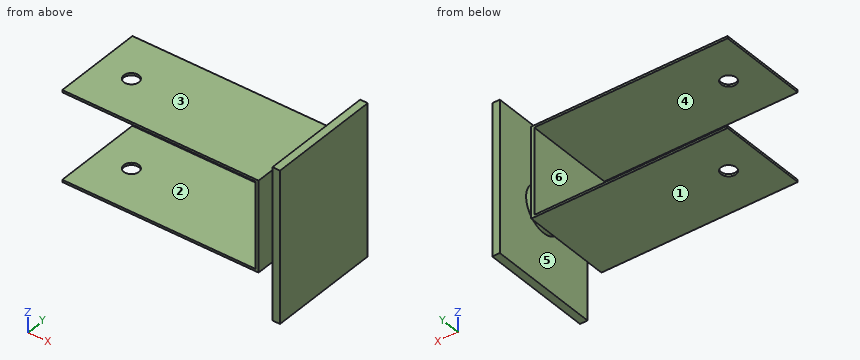
```python
from build123d import *

# Parameters (mm, degrees)
RESSALTO_EXTRUS_O1_DEPTH   = 60
CORTE_EXTRUS_O1_DEPTH      = 148.170653102
CORTE_EXTRUS_O1_DEPTH_BACK = 148.170653102
CORTE_EXTRUS_O2_DEPTH      = 148.170653102
CORTE_EXTRUS_O2_DEPTH_BACK = 148.170653102
ESBO_O5_W                  = 126
ESBO_O5_H                  = 57
ESBO_O6_W                  = 57
ESBO_O6_H                  = 60
CORTE_EXTRUS_O3_DEPTH      = 57
CORTE_EXTRUS_O4_DEPTH      = 148.170653102
CORTE_EXTRUS_O4_DEPTH_BACK = 57
ESBO_O7_R                  = 5
CORTE_EXTRUS_O5_DEPTH      = 148.170653102
CORTE_EXTRUS_O5_DEPTH_BACK = 148.170653102
ESBO_O8_W                  = 65.993133921
ESBO_O8_H                  = 60
ESBO_O13_R                 = 15
RESSALTO_EXTRUS_O2_DEPTH   = 15
ESBO_O14_W                 = 100
ESBO_O14_H                 = 75
RESSALTO_EXTRUS_O3_DEPTH   = 5


with BuildPart() as part:
    # Esboço1 → Ressalto-extrusão1 (new body)
    with BuildSketch(Plane.XY):
        with BuildLine():
            Line((65, 30), (-65, 30))
            Line((-65, 30), (-65, -30))
            Line((-65, -30), (65, -30))
            ThreePointArc((65, -30), (101.246012625, -22.148036763), (130.993133921, 0))
            ThreePointArc((130.993133921, 0), (101.246012625, 22.148036763), (65, 30))
        make_face()
    extrude(amount=RESSALTO_EXTRUS_O1_DEPTH)

    # Esboço3 → Corte-extrusão1 (cut, two sides: drawn at the far end of the back side and taken through both)
    with BuildSketch(Plane.XY.offset(-CORTE_EXTRUS_O1_DEPTH_BACK)):
        with BuildLine():
            Line((65, 25), (65, -25))
            ThreePointArc((65, -25), (88.305470739, -18.221231084), (104.339291624, 0))
            ThreePointArc((104.339291624, 0), (88.305470739, 18.221231084), (65, 25))
        make_face()
    extrude(amount=CORTE_EXTRUS_O1_DEPTH + CORTE_EXTRUS_O1_DEPTH_BACK, mode=Mode.SUBTRACT)

    # Esboço5 → Corte-extrusão2 (cut, two sides: drawn at the far end of the back side and taken through both)
    with BuildSketch(Plane(origin=(0, 0, 0), x_dir=(1, 0, 0), z_dir=(0, 1, 0)).offset(-CORTE_EXTRUS_O2_DEPTH_BACK)):
        with Locations((0, -30)):
            Rectangle(ESBO_O5_W, ESBO_O5_H)
    extrude(amount=CORTE_EXTRUS_O2_DEPTH + CORTE_EXTRUS_O2_DEPTH_BACK, mode=Mode.SUBTRACT)

    # Esboço6 → Corte-extrusão3 (cut)
    with BuildSketch(Plane(origin=(-63, 0, 0), x_dir=(0, 0, -1), z_dir=(1, 0, 0))):
        with Locations((-30, 0)):
            Rectangle(ESBO_O6_W, ESBO_O6_H)
    extrude(amount=-CORTE_EXTRUS_O3_DEPTH, mode=Mode.SUBTRACT)

    # Esboço7 → Corte-extrusão4 (cut, two sides: drawn at the far end of the back side and taken through both)
    with BuildSketch(Plane.XY.offset(-CORTE_EXTRUS_O4_DEPTH_BACK)):
        with Locations((-42.467037106, 0)):
            Circle(ESBO_O7_R)
    extrude(amount=CORTE_EXTRUS_O4_DEPTH + CORTE_EXTRUS_O4_DEPTH_BACK, mode=Mode.SUBTRACT)

    # Esboço8 → Corte-extrusão5 (cut, two sides: drawn at the far end of the back side and taken through both)
    with BuildSketch(Plane(origin=(0, 0, 0), x_dir=(1, 0, 0), z_dir=(0, 1, 0)).offset(-CORTE_EXTRUS_O5_DEPTH_BACK)):
        with Locations((97.996566961, -30)):
            Rectangle(ESBO_O8_W, ESBO_O8_H)
    extrude(amount=CORTE_EXTRUS_O5_DEPTH + CORTE_EXTRUS_O5_DEPTH_BACK, mode=Mode.SUBTRACT)

    # Esboço13 → Ressalto-extrusão2 (add)
    with BuildSketch(Plane(origin=(65, 0, 0), x_dir=(0, 0, -1), z_dir=(1, 0, 0))):
        with Locations((-30, 0)):
            Circle(ESBO_O13_R)
    extrude(amount=RESSALTO_EXTRUS_O2_DEPTH)

    # Esboço14 → Ressalto-extrusão3 (add)
    with BuildSketch(Plane(origin=(80, 0, 0), x_dir=(0, 0, -1), z_dir=(1, 0, 0))):
        with Locations((-30, 0)):
            Rectangle(ESBO_O14_W, ESBO_O14_H)
    extrude(amount=RESSALTO_EXTRUS_O3_DEPTH)


solid = part.part
```
Read the model definition and answer for the solid it produces. Units are mm, in the model's axes. Face numbers are marked on the shaded views. A direction names the side the tool comes from. Coordinates: 2 decimals unless noted, no trailing zeros. Write each loop counter-clockwise with the first axis right and the second up, starting at its lowest first coordinate (ties: lowest second). Pieces come first, ordered by that corner, then holes. Notation, with made-up numbers: (62.25, 8.5) -> (113.25, 8.5) arc R15 ccw to (113.25, 15.5) -> close; hole circle Ø2 at (69, 85). An arc over 180 degrees is marked (long way). Return JSON: item names as keys, results as strings.
1. Find the intervals of material crossed by line 1 along X through (y, z) = (0, 1); line 2 along Z through (x, y) = (15, -20); line 3 along X through (y, z) = (10, 18), in increasing order. Write a range as from..to.
Found:
{"line 1": "-65..-47.47, -37.47..65, 80..85", "line 2": "0..1.5, 58.5..60", "line 3": "63..65, 80..85"}
2. A tool of negligible diameter and unlimited length cuts with its end or side. For the marked faces 1, 2 and 3, from which of +Z, -Z, +X, -X, +Y, -Y can it reach the whole face along a straight path? Write none if from no direction.
Found:
{"face 1": "-Z, -X, +Y, -Y", "face 2": "-X, +Y, -Y", "face 3": "+Z, -X, +Y, -Y"}
3. A cutting plane is placed at A-A (z = 55). Determine the outline of the cut face in (x, y).
Found:
{"outline": "(63, -30) -> (65, -30) -> (65, 30) -> (63, 30) -> close; (80, -37.5) -> (85, -37.5) -> (85, 37.5) -> (80, 37.5) -> close"}
4. Determine the mould class of the marked faces 4, 5 and 6 for opening direction X: pulls with the +X half, pulls with the -X half, needs draft (parallel to the pull), parting line crosses it, or undercut.
Found:
{"face 4": "needs draft", "face 5": "undercut", "face 6": "pulls with the -X half"}
5. Each of these flat-tipped pins is pushed along its axis until it touches: P1, Ø1, axis at x = -28.5, y = -23, coming from the -Z side; P2, Ø12, axis at y = -7.5, z = 45, coming from the -X side; P3, Ø3, axis at x = 22, y = -25, coming from the +Z side. Where does it stop, or does it pass through?
Found:
{"P1": "z = 0", "P2": "x = 63", "P3": "z = 60"}
6. A cutting plane is placed at B-B (y = 0). Determine the outline of the cut face in (x, z).
Found:
{"outline": "(-65, 0) -> (-47.47, 0) -> (-47.47, 1.5) -> (-65, 1.5) -> close; (-65, 58.5) -> (-47.47, 58.5) -> (-47.47, 60) -> (-65, 60) -> close; (-37.47, 0) -> (65, 0) -> (65, 15) -> (80, 15) -> (80, -20) -> (85, -20) -> (85, 80) -> (80, 80) -> (80, 45) -> (65, 45) -> (65, 60) -> (-37.47, 60) -> (-37.47, 58.5) -> (63, 58.5) -> (63, 1.5) -> (-37.47, 1.5) -> close"}
7. A cutting plane is placed at D-D (y = 19.5). Determine the outline of the cut face in (x, z), and give its area (3 significant figures).
Found:
{"outline": "(-65, 0) -> (65, 0) -> (65, 60) -> (-65, 60) -> (-65, 58.5) -> (63, 58.5) -> (63, 1.5) -> (-65, 1.5) -> close; (80, -20) -> (85, -20) -> (85, 80) -> (80, 80) -> close", "area": "1,000 mm2"}
8. A cutting plane is placed at C-C (x = -40). Determine the outline of the cut face in (y, z).
Found:
{"outline": "(-30, 0) -> (-4.35, 0) -> (-4.35, 1.5) -> (-30, 1.5) -> close; (-30, 58.5) -> (-4.35, 58.5) -> (-4.35, 60) -> (-30, 60) -> close; (4.35, 0) -> (30, 0) -> (30, 1.5) -> (4.35, 1.5) -> close; (4.35, 58.5) -> (30, 58.5) -> (30, 60) -> (4.35, 60) -> close"}
